from build123d import *

# Parameters (mm, degrees)
EXTRUDE_1_DEPTH       = 1
HOLE_WIZARD_M41_D     = 4.5
HOLE_WIZARD_M41_DEPTH = 5
HOLE_WIZARD_M41_TIP   = 1.351936393
SKETCH_4_W            = 5
SKETCH_4_H            = 190
SKETCH_4_W_2          = 15
SKETCH_4_H_2          = 160
CUT_EXTRUDE_1_DEPTH   = 467.760109692
FILLET_1_R            = 5
HOLE_WIZARD_M31_D     = 3.4
HOLE_WIZARD_M31_DEPTH = 5
HOLE_WIZARD_M31_TIP   = 1.021463052


with BuildPart() as part:
    # Эскиз1 → Бобышка-Вытянуть1 (new body)
    with BuildSketch(Plane.XY):
        Polygon((55, 319), (55, 458), (0, 458), (0, 0), (55, 0), (55, 99), (90, 99), (90, 319), align=None)
    extrude(amount=EXTRUDE_1_DEPTH)

    # Отверстие с зазором M41
    with Locations(Plane.XY.offset(1)):
        with Locations((15, 20), (15, 72.25), (15, 124.5), (15, 176.75), (15, 229), (15, 281.25), (15, 333.5), (15, 385.75), (15, 438)):
            Hole(HOLE_WIZARD_M41_D / 2, depth=HOLE_WIZARD_M41_DEPTH)
            with Locations((0, 0, -(HOLE_WIZARD_M41_DEPTH + HOLE_WIZARD_M41_TIP / 2))):  # 118° drill point
                Cone(0, HOLE_WIZARD_M41_D / 2, HOLE_WIZARD_M41_TIP, mode=Mode.SUBTRACT)

    # Эскиз4 → Вырез-Вытянуть1 (cut, through all)
    with BuildSketch(Plane.XY.offset(1)):
        with Locations((80.5, 209)):
            Rectangle(SKETCH_4_W, SKETCH_4_H)
        with Locations((52.5, 209)):
            Rectangle(SKETCH_4_W_2, SKETCH_4_H_2)
    extrude(amount=-CUT_EXTRUDE_1_DEPTH, mode=Mode.SUBTRACT)

    # Скругление1
    fillet_1_edges = [part.edges().sort_by_distance(p)[0] for p in [
        (60, 289, 0.5),
        (60, 129, 0.5),
        (45, 129, 0.5),
        (45, 289, 0.5),
    ]]
    fillet(fillet_1_edges, radius=FILLET_1_R)

    # Отверстие с зазором M31
    with Locations(Plane.XY.offset(1)):
        with Locations((82, 106.5), (82, 311.5), (60, 106.5), (60, 311.5), (38, 106.5), (38, 311.5), (16, 106.5), (16, 311.5)):
            Hole(HOLE_WIZARD_M31_D / 2, depth=HOLE_WIZARD_M31_DEPTH)
            with Locations((0, 0, -(HOLE_WIZARD_M31_DEPTH + HOLE_WIZARD_M31_TIP / 2))):  # 118° drill point
                Cone(0, HOLE_WIZARD_M31_D / 2, HOLE_WIZARD_M31_TIP, mode=Mode.SUBTRACT)


solid = part.part
Here's how the part is built. I have some questions about the finished solid (model axes, mm). Round coordinates to 2 decimals unless told otherwise and drop trailing zeros. Loops run counter-clockwise (first coordinate to the right, second up) from the corner with the lowest first, then second, coordinate; pieces in that order, holes last.
1. If we section it at B-B on z = 0.3: Count the separate pieces of the cut face and the enclosed holes in it, plus the area to 3 significant figures.
Answer list:
separate pieces: 1
enclosed holes: 19
area: 29,300 mm2
2. For P1, Ø5, axis at x = 15, y = 20, coming from the +Z side; P2, Ø2.5, axis at x = 15, y = 281.25, coming from the +Z side, each with a flat end and sliding along its axis, tell me the tip position at first contact or that it passes through.
Answer list:
P1: stops at z = 1
P2: passes through
3. If we section it at C-C on y = 355.5: Write out the boundary of the cut face in (x, z), plus the area to 3 significant figures.
Answer list:
outline: (0, 0) - (55, 0) - (55, 1) - (0, 1) - close
area: 55.0 mm2
4. If I drill on line 1 along X through (y, z) = (162, 0.45); line 2 along X through (y, z) = (385.5, 0.75); line 3 along Y through (x, z) = (82.5, 0.85), over which ranges is the centre line in solid material (lowest first)?
Answer list:
line 1: x = 0 to 45, 60 to 78, 83 to 90
line 2: x = 0 to 12.76, 17.24 to 55
line 3: y = 99 to 104.88, 108.12 to 114, 304 to 309.88, 313.12 to 319
5. If we section it at A-A on y = 201.5: Write out the boundary of the cut face in (x, z), plus the area to 3 significant figures.
Answer list:
outline: (0, 0) - (45, 0) - (45, 1) - (0, 1) - close; (60, 0) - (78, 0) - (78, 1) - (60, 1) - close; (83, 0) - (90, 0) - (90, 1) - (83, 1) - close
area: 70.0 mm2
